Read the model definition and answer for the solid it produces. Units are mm, in the model's axes. Face numbers are marked on the shaded views. A direction names the side the tool comes from. Coordinates: 2 decimals unless noted, no trailing zeros. Loops run counter-clockwise (first coordinate to the right, second up) from the corner with the lowest first, then second, coordinate; pieces in that order, holes last. Notation, with made-up numbers: (27, 71.5) -> (72, 71.5) arc R12 ccw to (72, 84.5) -> close; hole circle Ø7 at (11.25, -10). An arc over 180 degrees is marked (long way). Answer as a JSON object with one key per item and string values. Group by question number.
1) Flat-ended cylindrical pins translate along their axes: P1, Ø8, axis at x = 7, z = 1.5, coming from the -Y side; P2, Ø5, axis at x = 53.5, z = 7, coming from the -Y side; P3, Ø12, axis at x = 42.5, y = -1, coming from the +Z side; P4, Ø2.5, axis at y = 0, z = -8.5, coming from the +X side. Find the tip coordinate at first contact, or state that the pin passes through.
2) Consider probe 1 along X at (y, z) = (-5, -9); probe 2 along X at (y, z) = (3.75, 5.75); probe 3 along Y at (x, z) = (48.85, -8.5). Determine where each line is inside the solid, lowest interval first. Write a range as [from, to].
3) Section B-B, the plane y = 9.75 is taken. Give the vertices of the cut face in (x, z).
4) Which of the six approach directions +Z, -Z, +X, -X, +Y, -Y give full straight-line access (tool end or side, diameter ignored) to the marked faces 1, 2 and 3?
5) Section D-D, the plane x = 48 is taken. Give the vertices of the cut face in (y, z), plus the area to 3 significant figures.
6) Section C-C, the plane z = 0 is taken. Give the vertices of the cut face in (x, y).
7) Section A-A, the plane z = 8 is taken. Give the vertices of the cut face in (x, y).
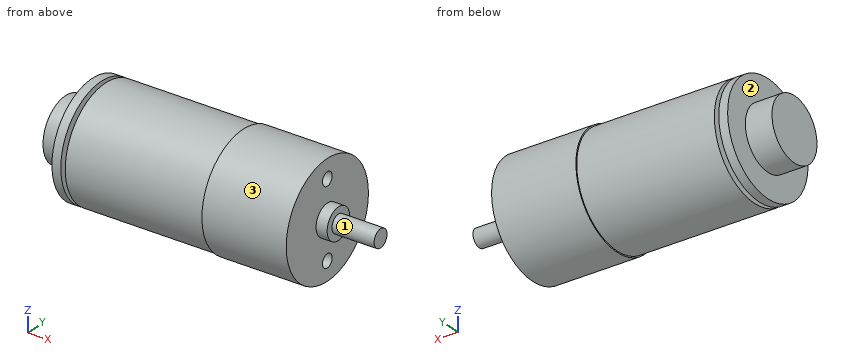
from build123d import *

# Parameters (mm, degrees)
SKETCH_1_R          = 12.5
EXTRUDE_1_DEPTH     = 31
SKETCH_2_R          = 12.76725859
EXTRUDE_2_DEPTH     = 19
SKETCH_3_R          = 3.5
EXTRUDE_3_DEPTH     = 2.5
SKETCH_4_R          = 2
EXTRUDE_4_DEPTH     = 9.5
EXTRUDE_START       = 1
SKETCH_5_R          = 12.5
EXTRUDE_5_DEPTH     = 2
SKETCH_6_R          = 1.579870025
EXTRUDE_6_DEPTH     = 4
SKETCH_7_R          = 7
EXTRUDE_7_DEPTH     = 6
SKETCH_8_R          = 1.5
CUT_EXTRUDE_1_DEPTH = 3


with BuildPart() as part:
    # Sketch 1 → Extrude 1 (new body)
    with BuildSketch(Plane(origin=(0, 0, 0), x_dir=(0, 0, -1), z_dir=(1, 0, 0))):
        Circle(SKETCH_1_R)
    extrude(amount=EXTRUDE_1_DEPTH)

    # Sketch 2 → Extrude 2 (add)
    with BuildSketch(Plane(origin=(31, 0, 0), x_dir=(0, 0, -1), z_dir=(1, 0, 0))):
        Circle(SKETCH_2_R)
    extrude(amount=EXTRUDE_2_DEPTH)

    # Sketch 3 → Extrude 3 (add)
    with BuildSketch(Plane(origin=(50, 0, 0), x_dir=(0, 0, -1), z_dir=(1, 0, 0))):
        Circle(SKETCH_3_R)
    extrude(amount=EXTRUDE_3_DEPTH)

    # Sketch 4 → Extrude 4 (add)
    with BuildSketch(Plane(origin=(52.5, 0, 0), x_dir=(0, 0, -1), z_dir=(1, 0, 0))):
        Circle(SKETCH_4_R)
    extrude(amount=EXTRUDE_4_DEPTH)



with BuildPart() as body_2:
    # Sketch 5 → Extrude 5 (new body)
    with BuildSketch(Plane.ZY.offset(EXTRUDE_START)):
        with Locations(Location((0, 0, 0), (0, 0, 180))):
            Circle(SKETCH_5_R)
    extrude(amount=EXTRUDE_5_DEPTH)


with BuildPart() as part_1:
    add(part.part)

    add(body_2.part)  # Extrude 6 merges body 2
    # Sketch 6 → Extrude 6 (add)
    with BuildSketch(Plane.ZY.offset(3)):
        Circle(SKETCH_6_R)
    extrude(amount=-EXTRUDE_6_DEPTH)

    # Sketch 7 → Extrude 7 (add)
    with BuildSketch(Plane.ZY.offset(3)):
        Circle(SKETCH_7_R)
    extrude(amount=EXTRUDE_7_DEPTH)

    # Sketch 8 → Cut-Extrude 1 (cut)
    with BuildSketch(Plane(origin=(50, 0, 0), x_dir=(0, 0, -1), z_dir=(1, 0, 0))):
        with Locations((8.5, 0)):
            Circle(SKETCH_8_R)
        with Locations(Location((-8.5, 0, 0), (0, 0, 180))):
            Circle(SKETCH_8_R)
    extrude(amount=-CUT_EXTRUDE_1_DEPTH, mode=Mode.SUBTRACT)


solid = part_1.part
Determined:
{
 "1": {"P1": "y = -12.5", "P2": "through", "P3": "z = 12.77", "P4": "x = 47"},
 "2": {"probe 1": "[-3, -1], [0, 50]", "probe 2": "[-9, -1], [0, 50]", "probe 3": "[-9.53, -1.5], [1.5, 9.53]"},
 "3": {"outline": "(-3, -7.82) -> (-1, -7.82) -> (-1, 7.82) -> (-3, 7.82) -> close; (0, -7.82) -> (31, -7.82) -> (31, -8.24) -> (50, -8.24) -> (50, 8.24) -> (31, 8.24) -> (31, 7.82) -> (0, 7.82) -> close"},
 "4": {"face 1": "+X", "face 2": "-X", "face 3": "+X, -X"},
 "5": {"outline": "circle Ø25.53 at (0, 0); hole circle Ø3 at (0, -8.5); hole circle Ø3 at (0, 8.5)", "area": "498 mm²"},
 "6": {"outline": "(-9, -7) -> (-3, -7) -> (-3, -12.5) -> (-1, -12.5) -> (-1, -1.58) -> (0, -1.58) -> (0, -12.5) -> (31, -12.5) -> (31, -12.77) -> (50, -12.77) -> (50, -3.5) -> (52.5, -3.5) -> (52.5, -2) -> (62, -2) -> (62, 2) -> (52.5, 2) -> (52.5, 3.5) -> (50, 3.5) -> (50, 12.77) -> (31, 12.77) -> (31, 12.5) -> (0, 12.5) -> (0, 1.58) -> (-1, 1.58) -> (-1, 12.5) -> (-3, 12.5) -> (-3, 7) -> (-9, 7) -> close"},
 "7": {"outline": "(-3, -9.6) -> (-1, -9.6) -> (-1, 9.6) -> (-3, 9.6) -> close; (0, -9.6) -> (31, -9.6) -> (31, -9.95) -> (50, -9.95) -> (50, -1.41) -> (47, -1.41) -> (47, 1.41) -> (50, 1.41) -> (50, 9.95) -> (31, 9.95) -> (31, 9.6) -> (0, 9.6) -> close"}
}
